Verification items for the finished model (mm, model axes). A direction names the side the tool comes from. Give positions to 0.01 mm unless a question says otherwise; leave off trailing zeros. Write each loop counter-clockwise with the first axis right and the second up, starting at its lowest first coordinate (ties: lowest second). Pieces come first, ordered by that corner, then holes. Notation, with made-up numbers: M 76,62.25 L 91,62.25 A27 ccw 91,87.25 Z; hole C -24.75,-20 d8. An arc over 180 degrees is marked long. Answer as a JSON object with one key per item and string values.
```python
from build123d import *

# Parameters (mm, degrees)
F1_DEPTH = 152.4
F3_DEPTH = 50.8
F5_DEPTH = 50.8
F6_R     = 5.07999


# Not quite as in the source:
# - a fillet or chamfer is up to 0.001 mm smaller than in the source, because OpenCascade refuses the exact size


with BuildPart() as f1:
    # F0 (on Front) → F1 (new body)
    with BuildSketch(Plane.XZ):
        Polygon((25.4, 35.56), (-25.4, 35.56), (-25.4, 22.86), (-12.7, 22.86), (-12.7, 0), (0, 0), (7.62, 0), (7.62, 7.62), (17.78, 7.62), (17.78, 12.7), (25.4, 12.7), align=None)
    extrude(amount=F1_DEPTH)

    # F2 (on face) → F3 (cut)
    with BuildSketch(Plane.YZ.offset(25.4)):
        Polygon((-116.84, 0), (-152.4, 35.56), (-152.4, 0), align=None)
    extrude(amount=-F3_DEPTH, mode=Mode.SUBTRACT)

    # F4 (on face) → F5 (cut)
    with BuildSketch(Plane.YZ.offset(25.4)):
        Polygon((0, 0), (0, 35.56), (-35.56, 0), align=None)
    extrude(amount=-F5_DEPTH, mode=Mode.SUBTRACT)

    # F6 (radius 5.08 in the source; OpenCascade refuses exactly that, so slightly less here)
    f6_edges = [f1.edges().sort_by_distance(p)[0] for p in [
        (17.78, -76.2, 7.62),
    ]]
    fillet(f6_edges, radius=F6_R)


solid = f1.part
```
1) Section check B-B on x = -10.5. Record the boundary of the cut face in (y, z).
Completed:
{"outline": "M -152.4,35.56 L -116.84,0 L -35.56,0 L 0,35.56 Z"}
2) Access from +Z, -Z, +X, -X, +Y, -Y to the whole of each face (thin tool, end or side, straight path). Record for faces 1 (the face through (10, -76, 7.62)), 2 (the face through (-3, -76, 0)), 3 (the face through (-12.7, -75, 12)).
Completed:
{"face 1": "-Z, +X, +Y, -Y", "face 2": "-Z, +X, -X, +Y, -Y", "face 3": "-Z, -X, +Y, -Y"}
3) Thickness scan on L1, parallel to X at y = -119.5, z = 5; L2, parallel to Z at x = -14, y = -45; L3, parallel to X at y = -32.5, z = 15.5. Record the ranges inside material, lowest first.
Completed:
{"L1": "x = -12.7 to 7.62", "L2": "z = 22.86 to 35.56", "L3": "x = -12.7 to 25.4"}
4) Go/stop test with flat-tipped pins: pin 1 (6 mm diameter, centred on x = 20, y = -72, fed in from -Z); pin 2 (8 mm diameter, centred on x = -0.5, z = 17, fed in from +Y); pin 3 (4 mm diameter, centred on y = -59.5, z = 16.5, fed in from -X). Record where each tip stops, or that it passes through.
Completed:
{"pin 1": "stops at z = 10", "pin 2": "stops at y = -14.56", "pin 3": "stops at x = -12.7"}
5) Section check C-C on z = 28.5. Record the boundary of the cut face in (x, y).
Completed:
{"outline": "M -25.4,-145.34 L 25.4,-145.34 L 25.4,-7.06 L -25.4,-7.06 Z"}
